```python
from build123d import *

# Parameters (mm, degrees)
SKETCH_1_R      = 1.6
EXTRUDE_2_DEPTH = 3


with BuildPart() as part:
    # 草图1 → 凸台-拉伸2 (new body)
    with BuildSketch(Plane(origin=(0, 0, 0), x_dir=(1, 0, 0), z_dir=(0, 1, 0))):
        Polygon((-61, 107), (-22.5, 107), (-22.5, 57), (2.5, 57), (2.5, 107), (61, 107), (69, 99), (69, -99), (61, -107), (-61, -107), (-69, -99), (-69, 99), align=None)
        with Locations(Location((60, 59, 0), (0, 0, 270))):
            Circle(SKETCH_1_R, mode=Mode.SUBTRACT)
        with Locations(Location((36, 59, 0), (0, 0, 270))):
            Circle(SKETCH_1_R, mode=Mode.SUBTRACT)
        with Locations(Location((60, 89, 0), (0, 0, 270))):
            Circle(SKETCH_1_R, mode=Mode.SUBTRACT)
        with Locations(Location((36, 89, 0), (0, 0, 270))):
            Circle(SKETCH_1_R, mode=Mode.SUBTRACT)
        with Locations(Location((-60, 89, 0), (0, 0, 270))):
            Circle(SKETCH_1_R, mode=Mode.SUBTRACT)
        with Locations(Location((-60, 59, 0), (0, 0, 270))):
            Circle(SKETCH_1_R, mode=Mode.SUBTRACT)
        with Locations(Location((-36, 89, 0), (0, 0, 270))):
            Circle(SKETCH_1_R, mode=Mode.SUBTRACT)
        with Locations(Location((-36, 59, 0), (0, 0, 270))):
            Circle(SKETCH_1_R, mode=Mode.SUBTRACT)
        with Locations(Location((60, -59, 0), (0, 0, 90))):
            Circle(SKETCH_1_R, mode=Mode.SUBTRACT)
        with Locations(Location((60, -89, 0), (0, 0, 90))):
            Circle(SKETCH_1_R, mode=Mode.SUBTRACT)
        with Locations(Location((36, -59, 0), (0, 0, 90))):
            Circle(SKETCH_1_R, mode=Mode.SUBTRACT)
        with Locations(Location((36, -89, 0), (0, 0, 90))):
            Circle(SKETCH_1_R, mode=Mode.SUBTRACT)
        with Locations(Location((-36, -59, 0), (0, 0, 90))):
            Circle(SKETCH_1_R, mode=Mode.SUBTRACT)
        with Locations(Location((-36, -89, 0), (0, 0, 90))):
            Circle(SKETCH_1_R, mode=Mode.SUBTRACT)
        with Locations(Location((-60, -59, 0), (0, 0, 90))):
            Circle(SKETCH_1_R, mode=Mode.SUBTRACT)
        with Locations(Location((-60, -89, 0), (0, 0, 90))):
            Circle(SKETCH_1_R, mode=Mode.SUBTRACT)
        with Locations(Location((44, 44, 0), (0, 0, 270))):
            Circle(SKETCH_1_R, mode=Mode.SUBTRACT)
        with Locations(Location((60, 49, 0), (0, 0, 270))):
            Circle(SKETCH_1_R, mode=Mode.SUBTRACT)
        with Locations(Location((60, -99, 0), (0, 0, 270))):
            Circle(SKETCH_1_R, mode=Mode.SUBTRACT)
        with Locations(Location((-44, 44, 0), (0, 0, 90))):
            Circle(SKETCH_1_R, mode=Mode.SUBTRACT)
        with Locations(Location((44, -44, 0), (0, 0, 90))):
            Circle(SKETCH_1_R, mode=Mode.SUBTRACT)
        with Locations(Location((-44, -44, 0), (0, 0, 270))):
            Circle(SKETCH_1_R, mode=Mode.SUBTRACT)
        with Locations(Location((-60, -99, 0), (0, 0, 90))):
            Circle(SKETCH_1_R, mode=Mode.SUBTRACT)
        with Locations(Location((-60, 49, 0), (0, 0, 90))):
            Circle(SKETCH_1_R, mode=Mode.SUBTRACT)
        with Locations(Location((24.656854249, 75.343145751, 0), (0, 0, 270))):
            Circle(SKETCH_1_R, mode=Mode.SUBTRACT)
        with Locations(Location((-25.25, 97.25, 0), (0, 0, 270))):
            Circle(SKETCH_1_R, mode=Mode.SUBTRACT)
        with Locations(Location((5.25, 97.25, 0), (0, 0, 90))):
            Circle(SKETCH_1_R, mode=Mode.SUBTRACT)
        with Locations(Location((-25.25, 66.75, 0), (0, 0, 270))):
            Circle(SKETCH_1_R, mode=Mode.SUBTRACT)
        with Locations(Location((5.25, 66.75, 0), (0, 0, 90))):
            Circle(SKETCH_1_R, mode=Mode.SUBTRACT)
        with Locations(Location((13.343145751, 75.343145751, 0), (0, 0, 270))):
            Circle(SKETCH_1_R, mode=Mode.SUBTRACT)
        with Locations(Location((13.343145751, 86.656854249, 0), (0, 0, 270))):
            Circle(SKETCH_1_R, mode=Mode.SUBTRACT)
        with Locations(Location((24.656854249, 86.656854249, 0), (0, 0, 270))):
            Circle(SKETCH_1_R, mode=Mode.SUBTRACT)
        with BuildLine():
            Line((-52.158528232, 30), (-52.158528232, -30))
            ThreePointArc((-52.158528232, -30), (-58.158528232, -36), (-64.158528232, -30))
            Line((-64.158528232, -30), (-64.158528232, 30))
            ThreePointArc((-64.158528232, 30), (-58.158528232, 36), (-52.158528232, 30))
        make_face(mode=Mode.SUBTRACT)
        with BuildLine():
            Line((52.158528232, 30), (52.158528232, -30))
            ThreePointArc((52.158528232, -30), (58.158528232, -36), (64.158528232, -30))
            Line((64.158528232, -30), (64.158528232, 30))
            ThreePointArc((64.158528232, 30), (58.158528232, 36), (52.158528232, 30))
        make_face(mode=Mode.SUBTRACT)
        with BuildLine():
            Line((-23.75, -48.403395609), (23.75, -48.403395609))
            ThreePointArc((23.75, -48.403395609), (29.75, -54.403395609), (23.75, -60.403395609))
            Line((23.75, -60.403395609), (-23.75, -60.403395609))
            ThreePointArc((-23.75, -60.403395609), (-29.75, -54.403395609), (-23.75, -48.403395609))
        make_face(mode=Mode.SUBTRACT)
        with BuildLine():
            Line((12.5, 56.262836439), (30.458741979, 56.262836439))
            ThreePointArc((30.458741979, 56.262836439), (34.208741979, 52.512836439), (30.458741979, 48.762836439))
            Line((30.458741979, 48.762836439), (12.5, 48.762836439))
            ThreePointArc((12.5, 48.762836439), (8.75, 52.512836439), (12.5, 56.262836439))
        make_face(mode=Mode.SUBTRACT)
    extrude(amount=EXTRUDE_2_DEPTH)


solid = part.part
```
For this review, take the finished solid that the model builds, in its own axes (mm). A direction names the side the tool comes from. Give positions to 0.01 mm unless a question says otherwise; leave off trailing zeros. Order: outer loops, then holes, each group sorted by start corner. A loop starts at its lowest first (then second) coordinate and runs counter-clockwise, first axis right, second up.
1) Insertion check: pin 1 (1.9 mm diameter, centred on x = 60, z = 59, fed in from +Y). The pin has a flat end and moves straight along its axis. Give the tip position at first contact, or say it passes through.
2) Take a section at B-B (x = 21). Give the boundary of the cut face in (y, z), then the cut area to 4 significant figures.
3) Take a section at A-A (x = -4). Give the boundary of the cut face in (y, z), then the cut area to 3 significant figures.
4) Take a section at C-C (y = 0.45). State how many separate pieces and enclosed holes the cut face has, then the cut area to 3 significant figures.
5) For faces 4 (the face through (58.03, 1.48, 36)), 5 (the face through (-65, 1, -103)), list the 3-axis set-ups (+Z, -Z, +X, -X, +Y, -Y) from which the entire face can be reached by the end or side of a thin tool; tool diameter is ignored.
6) The part is to be moulded in two halves that separate along X. For faces 1 (the face through (-65, 1, 103)), 2 (the face through (65, 1, -103)), 3 (the face through (58.3, 1.5, -36)), say which applies: released by +X, released by -X, zero draft, split by the parting line, or undercut.
7) Wall thickness on line 1 (X direction, y = 1.9, z = 14); line 2 (Z direction, x = 17, y = 1.65); line 3 (Z direction, x = 5, y = 0.35): over which ranges is each line inside the solid? List them lowest first.
Derived:
1. pin 1: passes through
2. outline: (0, -107) - (3, -107) - (3, -56.26) - (0, -56.26) - close; (0, -48.76) - (3, -48.76) - (3, 48.4) - (0, 48.4) - close; (0, 60.4) - (3, 60.4) - (3, 107) - (0, 107) - close
2. area: 583.5 mm2
3. outline: (0, -57) - (3, -57) - (3, 48.4) - (0, 48.4) - close; (0, 60.4) - (3, 60.4) - (3, 107) - (0, 107) - close
3. area: 456 mm2
4. separate pieces: 1
4. enclosed holes: 36
4. area: 25,400 mm2
5. face 4: +Y, -Y
5. face 5: -Z, -X, +Y, -Y
6. face 1: released by -X
6. face 2: released by +X
6. face 3: undercut
7. line 1: x = -69 to -64.16, -52.16 to 52.16, 64.16 to 69
7. line 2: z = -107 to -56.26, -48.76 to 48.4, 60.4 to 107
7. line 3: z = -107 to -98.83, -95.67 to -68.33, -65.17 to 48.4, 60.4 to 107
